Design review of the part built by this model. Coordinates are the model's own, in mm. Coordinates: 2 decimals unless noted, no trailing zeros. Loops run counter-clockwise (first coordinate to the right, second up) from the corner with the lowest first, then second, coordinate; pieces in that order, holes last. Notation, with made-up numbers: (12, 39.5) -> (27, 39.5) arc R31 cw to (27, 63.5) -> close; hole circle Ø7 at (28, 26.5). An arc over 180 degrees is marked (long way). Use CSV: the item, a comma, the result in double quotes.
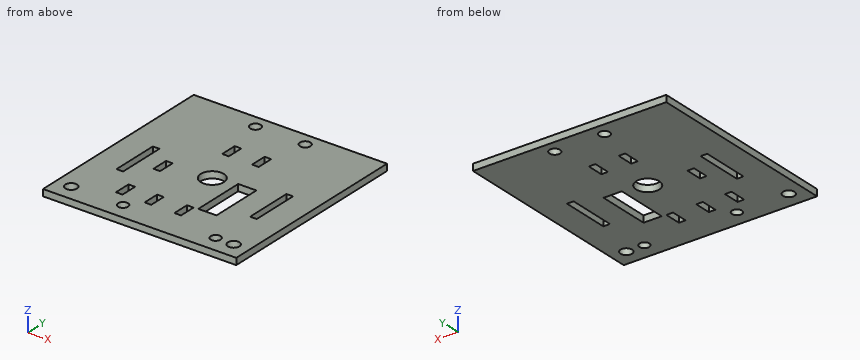
```python
from build123d import *

# Parameters (mm, degrees)
SKETCH1_R           = 3.5
SKETCH1_R_2         = 1.5
SKETCH1_R_3         = 2.5
SKETCH1_W           = 2
SKETCH1_H           = 5
SKETCH1_W_2         = 5.5
SKETCH1_H_2         = 15.95
SKETCH1_H_3         = 14.5
BOSS_EXTRUDE1_DEPTH = 2
SKETCH_5_W          = 53.3
SKETCH_5_H          = 62.979589089
CUT_EXTRUDE_1_DEPTH = 10
SKETCH_6_R          = 1.75
CUT_EXTRUDE_2_DEPTH = 10
SKETCH_7_W          = 2
SKETCH_7_H          = 65.797700214
EXTRUDE_1_DEPTH     = 2.5
SKETCH_8_W          = 2
SKETCH_8_H          = 65.797700214
EXTRUDE_2_DEPTH     = 2.5
SKETCH_9_W          = 58.3
SKETCH_9_H          = 2
EXTRUDE_3_DEPTH     = 2
SKETCH_10_W         = 58.3
SKETCH_10_H         = 5
CUT_EXTRUDE_3_DEPTH = 10
SKETCH_13_W         = 58.3
SKETCH_13_H         = 2.577289
CUT_EXTRUDE_4_DEPTH = 10
SKETCH_14_R         = 1.6
CUT_EXTRUDE_5_DEPTH = 10


with BuildPart() as part:
    # Sketch1 → Boss-Extrude1 (new body)
    with BuildSketch(Plane.XY):
        with BuildLine():
            Line((-25.65, 0), (25.65, 0))
            ThreePointArc((25.65, 0), (26.357106781, 0.292893219), (26.65, 1))
            Line((26.65, 1), (26.65, 123.726079281))
            Line((26.65, 123.726079281), (26.65, 128.777289303))
            Line((26.65, 128.777289303), (-26.65, 128.777289303))
            Line((-26.65, 128.777289303), (-26.65, 99.754415082))
            Line((-26.65, 99.754415082), (-26.65, 1))
            ThreePointArc((-26.65, 1), (-26.357106781, 0.292893219), (-25.65, 0))
        make_face()
        with Locations((0, 90)):
            Circle(SKETCH1_R, mode=Mode.SUBTRACT)
        with Locations((19.05, 66.1)):
            Circle(SKETCH1_R_2, mode=Mode.SUBTRACT)
        with Locations((-8.85, 66.1)):
            Circle(SKETCH1_R_2, mode=Mode.SUBTRACT)
        with Locations((-24.05, 15.3)):
            Circle(SKETCH1_R_2, mode=Mode.SUBTRACT)
        with Locations((24.15, 14)):
            Circle(SKETCH1_R_2, mode=Mode.SUBTRACT)
        with Locations((0, 34.3)):
            Circle(SKETCH1_R_3, mode=Mode.SUBTRACT)
        with Locations((4.5, 103.75)):
            Rectangle(SKETCH1_W, SKETCH1_H, mode=Mode.SUBTRACT)
        with Locations((9.55, 83.375)):
            Rectangle(SKETCH1_W_2, SKETCH1_H_2, mode=Mode.SUBTRACT)
        with Locations((20.15, 87)):
            Rectangle(SKETCH1_W, SKETCH1_H_3, mode=Mode.SUBTRACT)
        with Locations((4.5, 72.75)):
            Rectangle(SKETCH1_W, SKETCH1_H, mode=Mode.SUBTRACT)
        with Locations((-4.5, 72.75)):
            Rectangle(SKETCH1_W, SKETCH1_H, mode=Mode.SUBTRACT)
        with Locations((-20.15, 87)):
            Rectangle(SKETCH1_W, SKETCH1_H_3, mode=Mode.SUBTRACT)
        with Locations((-4.5, 103.75)):
            Rectangle(SKETCH1_W, SKETCH1_H, mode=Mode.SUBTRACT)
        with Locations((-13.15, 72.75)):
            Rectangle(SKETCH1_W, SKETCH1_H, mode=Mode.SUBTRACT)
        with Locations((-13.15, 87.75)):
            Rectangle(SKETCH1_W, SKETCH1_H, mode=Mode.SUBTRACT)
        Polygon((-20, 34.3), (-20, 36.05), (-7, 36.05), (-7, 34.3), (-7, 32.55), (-20, 32.55), align=None, mode=Mode.SUBTRACT)
        Polygon((-5.232050808, 39.362177826), (-15.732050808, 57.548711306), (-12.267949192, 59.548711306), (-1.767949192, 41.362177826), align=None, mode=Mode.SUBTRACT)
        Polygon((1.767949192, 41.362177826), (5.232050808, 39.362177826), (15.732050808, 57.548711306), (12.267949192, 59.548711306), align=None, mode=Mode.SUBTRACT)
        Polygon((7, 34.3), (7, 32.55), (20, 32.55), (20, 34.3), (20, 36.05), (7, 36.05), align=None, mode=Mode.SUBTRACT)
        Polygon((-1.767949192, 27.237822174), (-5.232050808, 29.237822174), (-15.732050808, 11.051288694), (-12.267949192, 9.051288694), align=None, mode=Mode.SUBTRACT)
        Polygon((15.732050808, 11.051288694), (12.267949192, 9.051288694), (1.767949192, 27.237822174), (5.232050808, 29.237822174), align=None, mode=Mode.SUBTRACT)
    extrude(amount=BOSS_EXTRUDE1_DEPTH)

    # 草图5 → 切除-拉伸1 (cut)
    with BuildSketch(Plane(origin=(0, 0, 0), x_dir=(-1, 0, 0), z_dir=(0, 0, -1))):
        with Locations((0, 31.489794545)):
            Rectangle(SKETCH_5_W, SKETCH_5_H)
    extrude(amount=-CUT_EXTRUDE_1_DEPTH, mode=Mode.SUBTRACT)

    # 草图6 → 切除-拉伸2 (cut)
    with BuildSketch(Plane.XY.offset(2)):
        with Locations((-24.5, 66.1)):
            Circle(SKETCH_6_R)
        with Locations((24.5, 66.1)):
            Circle(SKETCH_6_R)
    extrude(amount=-CUT_EXTRUDE_2_DEPTH, mode=Mode.SUBTRACT)

    # 草图7 → 凸台-拉伸1 (add)
    with BuildSketch(Plane(origin=(26.65, 0, 0), x_dir=(0, 0, -1), z_dir=(1, 0, 0))):
        with Locations((-1, 95.878439196)):
            Rectangle(SKETCH_7_W, SKETCH_7_H)
    extrude(amount=EXTRUDE_1_DEPTH)

    # 草图8 → 凸台-拉伸2 (add)
    with BuildSketch(Plane.ZY.offset(26.65)):
        with Locations((1, 95.878439196)):
            Rectangle(SKETCH_8_W, SKETCH_8_H)
    extrude(amount=EXTRUDE_2_DEPTH)

    # 草图9 → 凸台-拉伸3 (add)
    with BuildSketch(Plane.XZ.offset(-62.979589089)):
        with Locations((0, 1)):
            Rectangle(SKETCH_9_W, SKETCH_9_H)
    extrude(amount=EXTRUDE_3_DEPTH)

    # 草图10 → 切除-拉伸3 (cut)
    with BuildSketch(Plane.XY.offset(2)):
        with Locations((0, 126.277289303)):
            Rectangle(SKETCH_10_W, SKETCH_10_H)
    extrude(amount=-CUT_EXTRUDE_3_DEPTH, mode=Mode.SUBTRACT)

    # 草图13 → 切除-拉伸4 (cut)
    with BuildSketch(Plane.XY.offset(2)):
        with Locations((0, 122.488644803)):
            Rectangle(SKETCH_13_W, SKETCH_13_H)
    extrude(amount=-CUT_EXTRUDE_4_DEPTH, mode=Mode.SUBTRACT)

    # 草图14 → 切除-拉伸5 (cut)
    with BuildSketch(Plane.XY.offset(2)):
        with Locations((-7.5, 117.200000303)):
            Circle(SKETCH_14_R)
        with Locations((7.5, 117.200000303)):
            Circle(SKETCH_14_R)
    extrude(amount=-CUT_EXTRUDE_5_DEPTH, mode=Mode.SUBTRACT)


solid = part.part
```
Item 1: Add section C-C (y = 105). Give the boundary of the cut face in (x, z), then the cut area to 3 significant figures.
Checked values:
outline,"(-29.15, 0) -> (-5.5, 0) -> (-5.5, 2) -> (-29.15, 2) -> close; (-3.5, 0) -> (3.5, 0) -> (3.5, 2) -> (-3.5, 2) -> close; (5.5, 0) -> (29.15, 0) -> (29.15, 2) -> (5.5, 2) -> close"
area,"109 mm^2"
Item 2: To check wall thickness, follow line 1 along X through (y, z) = (66.1, 0.9); line 2 along Y through (x, z) = (7.5, 0.6); line 3 along Y through (x, z) = (-21, 1.15). State the ranges of each line that lie inside material, in increasing order.
Checked values:
line 1,"-29.15 to -26.25, -22.75 to -10.35, -7.35 to 17.55, 20.55 to 22.75, 26.25 to 29.15"
line 2,"60.98 to 75.4, 91.35 to 115.6, 118.8 to 121.2"
line 3,"60.98 to 79.75, 94.25 to 121.2"
Item 3: Add section B-B (y = 66.1). Give the boundary of the cut face in (x, z), then the cut area to 3 significant figures.
Checked values:
outline,"(-29.15, 0) -> (-26.25, 0) -> (-26.25, 2) -> (-29.15, 2) -> close; (-22.75, 0) -> (-10.35, 0) -> (-10.35, 2) -> (-22.75, 2) -> close; (-7.35, 0) -> (17.55, 0) -> (17.55, 2) -> (-7.35, 2) -> close; (20.55, 0) -> (22.75, 0) -> (22.75, 2) -> (20.55, 2) -> close; (26.25, 0) -> (29.15, 0) -> (29.15, 2) -> (26.25, 2) -> close"
area,"90.6 mm^2"
Item 4: Clearance check with a flat-ended pin moving along its axis: pin 1 (3 mm diameter, centred on x = -24.5, y = 66.1, fed in from -Z). State where the tip first meets the part, or that it passes through.
Checked values:
pin 1,"through"
Item 5: Add section D-D (y = 72.5). Give the boundary of the cut face in (x, z).
Checked values:
outline,"(-29.15, 0) -> (-14.15, 0) -> (-14.15, 2) -> (-29.15, 2) -> close; (-12.15, 0) -> (-5.5, 0) -> (-5.5, 2) -> (-12.15, 2) -> close; (-3.5, 0) -> (3.5, 0) -> (3.5, 2) -> (-3.5, 2) -> close; (5.5, 0) -> (29.15, 0) -> (29.15, 2) -> (5.5, 2) -> close"
Item 6: Add section A-A (x = 24.5). Give the boundary of the cut face in (y, z).
Checked values:
outline,"(60.98, 0) -> (64.35, 0) -> (64.35, 2) -> (60.98, 2) -> close; (67.85, 0) -> (121.2, 0) -> (121.2, 2) -> (67.85, 2) -> close"
